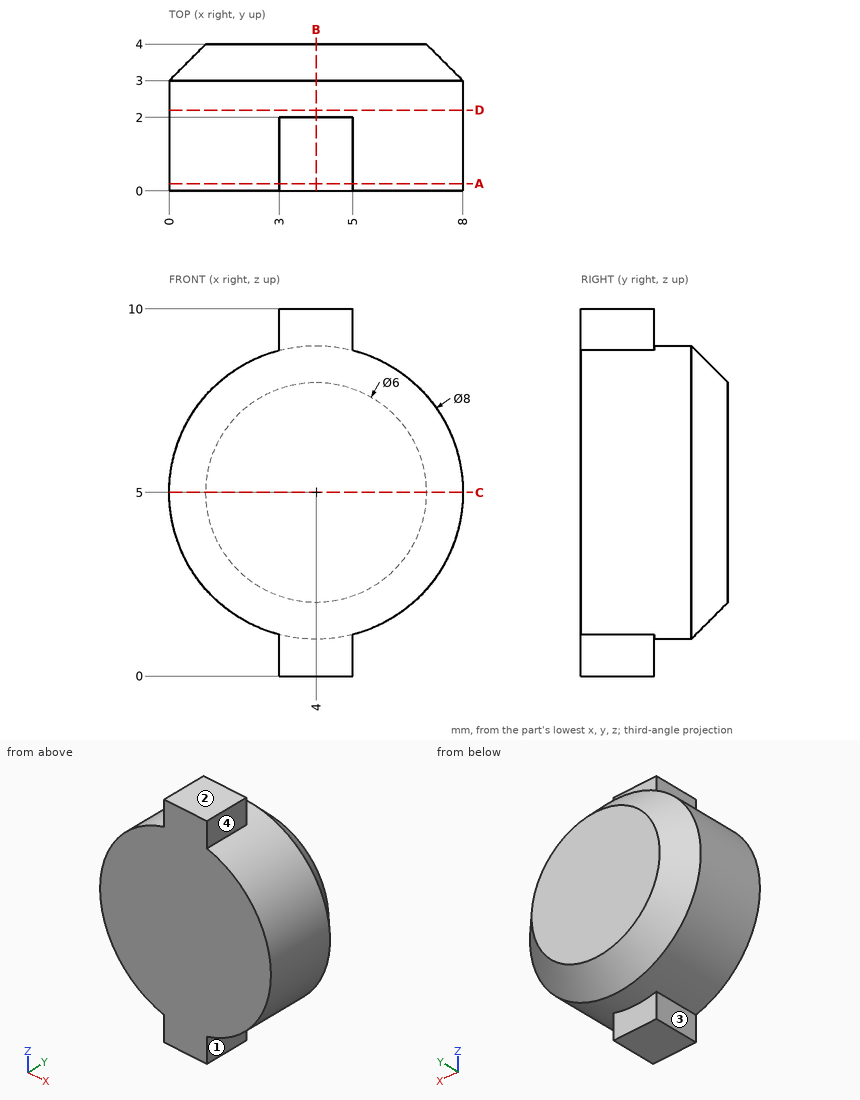
Answer from the drawing. Dimensions are ordinates in mm from the lowest x, y and z of the part. A direction names the side the tool comes from. Round coordinates to 2 decimals unless told otherwise and drop trailing zeros. Order: outer loops, then holes, each group sorted by start corner. A loop starts at its lowest first (then second) coordinate and runs counter-clockwise, first axis right, second up.
1) For the marked faces 1, 2, 3 and 4, determine the directions among +Z, -Z, +X, -X, +Y, -Y from which every point of the face is accessible in a straight line to the end or side of a thin tool.
2) Flat-ended cylindrical pins translate along their axes: pin 1 (0.6 mm diameter, centred on x = 4, z = 1, fed in from +Y); pin 2 (1.2 mm diameter, centred on y = 1, z = 1, fed in from -X); pin 3 (0.6 mm diameter, centred on y = 1, z = 0.5, fed in from +X). Find the tip coordinate at first contact, or state that the pin passes through.
3) The part is cut by section A-A on y = 0.2. Write down the section's boundary in (x, z).
4) The part is cut by section C-C on z = 5. Write down the section's boundary in (x, y), plus the area to 3 significant figures.
5) The part is cut by section D-D on y = 2.2. Write down the section's boundary in (x, z).
6) Straight lines are drawn through the part: L1, parallel to X at y = 1.7, z = 0.5; L2, parallel to X at y = 3.7, z = 2; L3, parallel to Z at x = 3, y = 3.1. For each, find the intervals that lie inside material, in ascending order.
7) The part is cut by section B-B on x = 4. Write down the section's boundary in (y, z).
Resolved:
1. face 1: -Z, +X, +Y, -Y
1. face 2: +Z, +X, -X, +Y, -Y
1. face 3: -Z, -X, +Y, -Y
1. face 4: +Z, +X, +Y, -Y
2. pin 1: stops at y = 3.3
2. pin 2: stops at x = 1.89
2. pin 3: stops at x = 5
3. outline: (3, 0) - (5, 0) - (5, 1.13) arc R4 ccw to (5, 8.87) - (5, 10) - (3, 10) - (3, 8.87) arc R4 ccw to (3, 1.13) - close
4. outline: (0, 0) - (8, 0) - (8, 3) - (7, 4) - (1, 4) - (0, 3) - close
4. area: 31.0 mm2
5. outline: circle Ø8 at (4, 5)
6. L1: x = 3 to 5
6. L2: x = 2.63 to 5.37
6. L3: z = 1.23 to 8.77
7. outline: (0, 0) - (2, 0) - (2, 1) - (3, 1) - (4, 2) - (4, 8) - (3, 9) - (2, 9) - (2, 10) - (0, 10) - close
